```python
from build123d import *

# Parameters (mm, degrees)
F0_R     = 14
F1_DEPTH = 2
F2_DEPTH = 2.5
F3_DEPTH = 3
F5_DEPTH = 0.5
F7_DEPTH = 2


# Not quite as in the source:
# - a feature names something its author has since deleted; it is built from what else it names


with BuildPart() as f1:
    # F0 (on Top) → F1 (new body)
    with BuildSketch(Plane.XY):
        with BuildLine():
            Line((18, -18), (18, 0))
            ThreePointArc((18, 0), (12.7279220614, 12.7279220614), (0, 18))
            ThreePointArc((0, 18), (-12.7279220614, 12.7279220614), (-18, 0))
            ThreePointArc((-18, 0), (-12.7279220614, -12.7279220614), (0, -18))
            Line((0, -18), (18, -18))
        make_face()
        Circle(F0_R, mode=Mode.SUBTRACT)
    extrude(amount=F1_DEPTH)

    # F0 (on Top) → F2 (join)
    with BuildSketch(Plane.XY):
        with BuildLine():
            Line((18, -18), (18, 0))
            ThreePointArc((18, 0), (12.7279220614, 12.7279220614), (0, 18))
            ThreePointArc((0, 18), (-12.7279220614, 12.7279220614), (-18, 0))
            ThreePointArc((-18, 0), (-12.7279220614, -12.7279220614), (0, -18))
            Line((0, -18), (18, -18))
        make_face()
        Circle(F0_R, mode=Mode.SUBTRACT)
        Circle(F0_R)
        with BuildLine():
            ThreePointArc((-4.1139610307, -6.3639610307), (-8.4426899788, -7.2249987535), (-4.772970773, -4.772970773))
            ThreePointArc((-4.772970773, -4.772970773), (-4.2852320825, -5.5029233079), (-4.1139610307, -6.3639610307))
        make_face(mode=Mode.SUBTRACT)
        with BuildLine():
            ThreePointArc((2.8284271247, 2.8284271247), (3.69551813, 1.5307337295), (4, 0))
            ThreePointArc((4, 0), (1.5307337295, -3.69551813), (-2.8284271247, -2.8284271247))
            ThreePointArc((-2.8284271247, -2.8284271247), (-3.69551813, 1.5307337295), (0, 4))
            ThreePointArc((0, 4), (1.5307337295, 3.69551813), (2.8284271247, 2.8284271247))
        make_face(mode=Mode.SUBTRACT)
        with BuildLine():
            ThreePointArc((8.6139610307, 6.3639610307), (7.2249987535, 4.2852320825), (4.772970773, 4.772970773))
            ThreePointArc((4.772970773, 4.772970773), (5.5029233079, 8.4426899788), (8.6139610307, 6.3639610307))
        make_face(mode=Mode.SUBTRACT)
        with BuildLine():
            ThreePointArc((-2.8284271247, -2.8284271247), (1.5307337295, -3.69551813), (4, 0))
            Line((4, 0), (0, 0))
            Line((0, 0), (-2.8284271247, -2.8284271247))
        make_face()
        with BuildLine():
            Line((0, 0), (2.8284271247, 2.8284271247))
            ThreePointArc((2.8284271247, 2.8284271247), (1.5307337295, 3.69551813), (0, 4))
            Line((0, 4), (0, 0))
        make_face()
        with BuildLine():
            ThreePointArc((0, 4), (-3.69551813, 1.5307337295), (-2.8284271247, -2.8284271247))
            Line((-2.8284271247, -2.8284271247), (0, 0))
            Line((0, 0), (0, 4))
        make_face()
        with BuildLine():
            Line((0, 0), (4, 0))
            ThreePointArc((4, 0), (3.69551813, 1.5307337295), (2.8284271247, 2.8284271247))
            Line((2.8284271247, 2.8284271247), (0, 0))
        make_face()
    extrude(amount=-F2_DEPTH)

    # F0 (on Top) → F3 (cut)
    with BuildSketch(Plane.XY):
        with BuildLine():
            ThreePointArc((-2.8284271247, -2.8284271247), (1.5307337295, -3.69551813), (4, 0))
            Line((4, 0), (0, 0))
            Line((0, 0), (-2.8284271247, -2.8284271247))
        make_face()
        with BuildLine():
            Line((0, 0), (4, 0))
            ThreePointArc((4, 0), (3.69551813, 1.5307337295), (2.8284271247, 2.8284271247))
            Line((2.8284271247, 2.8284271247), (0, 0))
        make_face()
        with BuildLine():
            Line((0, 0), (2.8284271247, 2.8284271247))
            ThreePointArc((2.8284271247, 2.8284271247), (1.5307337295, 3.69551813), (0, 4))
            Line((0, 4), (0, 0))
        make_face()
        with BuildLine():
            ThreePointArc((0, 4), (-3.69551813, 1.5307337295), (-2.8284271247, -2.8284271247))
            Line((-2.8284271247, -2.8284271247), (0, 0))
            Line((0, 0), (0, 4))
        make_face()
    extrude(amount=-F3_DEPTH, mode=Mode.SUBTRACT)

    # F4 (on face) → F5 (cut)
    with BuildSketch(Plane(origin=(0, 0, -2.5), x_dir=(1, 0, 0), z_dir=(0, 0, -1))):
        Polygon((4.2426406871, -4.2426406871), (0, 0), (-4.2426406871, 4.2426406871), (-16.9705627485, -8.4852813742), (-8.4852813742, -16.9705627485), align=None)
        Polygon((8.4852813742, 0), (0, 0), (4.2426406871, -4.2426406871), align=None)
        with BuildLine():
            Line((-2.8284271247, 2.8284271247), (0, 0))
            Line((0, 0), (4, 0))
            ThreePointArc((4, 0), (1.5307337295, 3.69551813), (-2.8284271247, 2.8284271247))
        make_face()
        with BuildLine():
            Line((-4.2426406871, 4.2426406871), (-2.8284271247, 2.8284271247))
            ThreePointArc((-2.8284271247, 2.8284271247), (1.5307337295, 3.69551813), (4, 0))
            Line((4, 0), (8.4852813742, 0))
            Line((8.4852813742, 0), (18, 9.5147186258))
            Line((18, 9.5147186258), (18, 18))
            Line((18, 18), (9.5147186258, 18))
            Line((9.5147186258, 18), (-4.2426406871, 4.2426406871))
        make_face()
    extrude(amount=-F5_DEPTH, mode=Mode.SUBTRACT)

    # F6 (on face) → F7 (cut)
    with BuildSketch(Plane.XY.offset(2)):
        with BuildLine():
            Line((5, -9), (0, -9))
            Line((0, -9), (0, -14))
            ThreePointArc((0, -14), (2.542267135, -13.7672392953), (5, -13.0766968306))
            Line((5, -13.0766968306), (5, -9))
        make_face()
        with BuildLine():
            Line((0, -14), (0, -9))
            Line((0, -9), (-5, -9))
            Line((-5, -9), (-5, -13.0766968306))
            ThreePointArc((-5, -13.0766968306), (-2.542267135, -13.7672392953), (0, -14))
        make_face()
        with BuildLine():
            Line((5, -18), (0, -18))
            ThreePointArc((0, -18), (-2.5249657043, -17.8220242451), (-5, -17.2916164658))
            Line((-5, -17.2916164658), (-5, -19))
            Line((-5, -19), (5, -19))
            Line((5, -19), (5, -18))
        make_face()
        with BuildLine():
            ThreePointArc((5, -13.0766968306), (2.542267135, -13.7672392953), (0, -14))
            Line((0, -14), (0, -18))
            Line((0, -18), (5, -18))
            Line((5, -18), (5, -13.0766968306))
        make_face()
        with BuildLine():
            Line((0, -18), (0, -14))
            ThreePointArc((0, -14), (-2.542267135, -13.7672392953), (-5, -13.0766968306))
            Line((-5, -13.0766968306), (-5, -17.2916164658))
            ThreePointArc((-5, -17.2916164658), (-2.5249657043, -17.8220242451), (0, -18))
        make_face()
    extrude(amount=-F7_DEPTH, mode=Mode.SUBTRACT)


solid = f1.part
```
Input: part model. Units: mm. Frame: model coordinates. A direction names the side the tool comes from. Give positions to 0.01 mm unless a question says otherwise; leave off trailing zeros. Order: outer loops, then holes, each group sorted by start corner. A loop starts at its lowest first (then second) coordinate and runs counter-clockwise, first axis right, second up.
1. Pin query (flat end, axial travel): pin 1 Ø1.5 at (y, z) = (-11.5, 0.5) entering from -X; pin 2 Ø6 at (x, y) = (4, -6.5) entering from +Z; pin 3 Ø2 at (y, z) = (-14.5, 1.5) entering from -X. Return the tip coordinate at first contact, or that it passes through.
Computed:
pin 1: stops at x = -14.44
pin 2: stops at z = 0
pin 3: stops at x = -11.91
2. Line query: probe 1 along Z at (x, y) = (1, 6); probe 2 along Y at (x, z) = (-7, 0.55); probe 3 along X at (y, z) = (-1, 1.65). Output: solid intervals per line, ascending.
Computed:
probe 1: z = -2 to 0
probe 2: y = -16.58 to -12.12, 12.12 to 16.58
probe 3: x = -17.97 to -13.96, 13.96 to 18
3. Cut plane D-D (x = 6.5). Return loops of the section in (y, z), and give its area (3 significant figures).
Computed:
outline: (-18, -2.5) - (-14.99, -2.5) - (-14.99, -2) - (1.99, -2) - (1.99, -2.5) - (4.12, -2.5) - (4.12, 0) - (-12.4, 0) - (-12.4, 2) - (-18, 2) - close; (8.61, -2.5) - (16.79, -2.5) - (16.79, 2) - (12.4, 2) - (12.4, 0) - (8.61, 0) - close
area: 87.2 mm2
4. Cut plane A-A (z = -0.9). Return loops of the section in (x, y), and give its area (3 significant figures).
Computed:
outline: (0, -18) - (18, -18) - (18, 0) arc R18 ccw (long way) to start; hole circle Ø4.5 at (-6.36, -6.36); hole circle Ø8 at (0, 0); hole circle Ø4.5 at (6.36, 6.36)
area: 1,010 mm2
5. Cut plane B-B (x = 0.5). Return loops of the section in (y, z).
Computed:
outline: (-18, -2.5) - (-8.99, -2.5) - (-8.99, -2) - (-3.97, -2) - (-3.97, 0) - (-18, 0) - close; (3.97, -2) - (7.99, -2) - (7.99, -2.5) - (17.99, -2.5) - (17.99, 2) - (13.99, 2) - (13.99, 0) - (3.97, 0) - close
6. Set-up query: faces 1 (the face through (0.54, 13.99, 0.99)), 2 (the face through (-5, -15, 1)), 3 (the face through (4.4, -1.1, -2)). Return all of +Z, -Z, +X, -X, +Y, -Y with unobstructed straight access to the full face (end or side cutting, diameter ignored); none if empty.
Computed:
face 1: +Z
face 2: +Z, -Y
face 3: -Z
7. Draft query along Y for faces 4 (the face through (0, -5, 0)), 5 (the face through (9, -18, 0)), 6 (the face through (5, -16, 1)). Return one class per face: released by +Y, released by -Y, zero draft, split by the parting line, or undercut.
Computed:
face 4: undercut
face 5: released by -Y
face 6: zero draft
8. Cut plane C-C (x = -12). Return loops of the section in (y, z), and give its area (3 significant figures).
Computed:
outline: (-13.42, -2.5) - (3.51, -2.5) - (3.51, -2) - (13.42, -2) - (13.42, 2) - (7.21, 2) - (7.21, 0) - (-7.21, 0) - (-7.21, 2) - (-13.42, 2) - close
area: 87.0 mm2
